Check sheet for the modelled part. Datum: model origin and axes. Units: mm. A direction names the side the tool comes from. Round coordinates to 2 decimals unless told otherwise and drop trailing zeros. Loops run counter-clockwise (first coordinate to the right, second up) from the corner with the lowest first, then second, coordinate; pieces in that order, holes last. Notation, with made-up numbers: (46, 60) - (89, 60) arc R26 ccw to (89, 76) - close; hole circle Ø2 at (14, 61). An arc over 180 degrees is marked (long way). Put each result on its own line as item: value. Start each with the question number.
Item 1: Gauge pin test, flat ends, axial feed: pin 1 Ø1.5 at (x, y) = (1.5, 10) entering from -Z; pin 2 Ø12 at (y, z) = (3.5, 5.5) entering from -X; pin 3 Ø1.5 at (x, y) = (1, -4.5) entering from +Z; pin 4 Ø1 at (x, z) = (1.5, -12.5) entering from -Y. Record the tip position at first contact, or that the pin passes through.
Item 2: Draft check along Z on faces 1 (the flat face through (0, 0, -4)), 2 (the cylindrical face through (1.528, 20.147, 2.645)), 3 (the cylindrical face through (1.53, 7.79, -13.1)). Enter one of: pulls with the +Z half, pulls with the -Z half, needs draft (parallel to the pull), parting line crosses it, or undercut.
Item 3: Section check B-B, the plane z = 0. Record the cut outline in (x, y).
Item 4: Tool access check on faces 4 (the flat face through (3.099, 0, -4)), 5 (the flat face through (2, 10, 1.905)). Record the directions out of +Z, -Z, +X, -X, +Y, -Y that give a thin tool (end or side, any length) a straight path to the whole face; none if there is none.
Item 5: Section check C-C, the plane z = 13.5. Record the cut outline in (x, y).
Item 6: Material ranges on line 1 along Y through (x, z) = (1.3, -7); line 2 along Z through (x, y) = (0.85, 7.5) (3 decimals); line 3 along Y through (x, z) = (1.05, 8.5), recorded low to high.
Item 7: Section check D-D, the plane y = 13. Record the cut outline in (x, z) (3 decimals).
Item 8: Section check A-A, the plane x = 1.7. Record the cut outline in (y, z) (1 decimal).
from build123d import *

# Parameters (mm, degrees)
SKETCH2_R           = 20.32
SKETCH2_R_2         = 1.0795
BOSS_EXTRUDE5_DEPTH = 3.0988


with BuildPart() as part:
    # Sketch2 → Boss-Extrude5 (new body)
    with BuildSketch(Plane(origin=(0, 0, 0), x_dir=(0, 0, -1), z_dir=(1, 0, 0))):
        Circle(SKETCH2_R)
        with BuildLine():
            Line((-12.142210048, -9.210012766), (-3.125861344, -4.004421414))
            ThreePointArc((-3.125861344, -4.004421414), (0, -5.08), (3.125861344, -4.004421414))
            Line((3.125861344, -4.004421414), (12.142210048, -9.210012766))
            ThreePointArc((12.142210048, -9.210012766), (0, -15.24), (-12.142210048, -9.210012766))
        make_face(mode=Mode.SUBTRACT)
        with BuildLine():
            ThreePointArc((-14.047210048, -5.910455977), (-13.198227154, 7.62), (-1.905, 15.120468743))
            Line((-1.905, 15.120468743), (-1.905, 4.709286039))
            ThreePointArc((-1.905, 4.709286039), (-4.399409051, 2.54), (-5.030861344, -0.704864625))
            Line((-5.030861344, -0.704864625), (-14.047210048, -5.910455977))
        make_face(mode=Mode.SUBTRACT)
        Circle(SKETCH2_R_2, mode=Mode.SUBTRACT)
        with BuildLine():
            Line((1.905, 4.709286039), (1.905, 15.120468743))
            ThreePointArc((1.905, 15.120468743), (13.198227154, 7.62), (14.047210048, -5.910455977))
            Line((14.047210048, -5.910455977), (5.030861344, -0.704864625))
            ThreePointArc((5.030861344, -0.704864625), (4.399409051, 2.54), (1.905, 4.709286039))
        make_face(mode=Mode.SUBTRACT)
    extrude(amount=BOSS_EXTRUDE5_DEPTH)


solid = part.part
Check result:
1. pin 1: z = -18.09
1. pin 2: x = 0
1. pin 3: z = 19.97
1. pin 4: y = -16.4
2. face 1: needs draft
2. face 2: parting line crosses it
2. face 3: undercut
3. outline: (0, -20.32) - (3.1, -20.32) - (3.1, -15.24) - (0, -15.24) - close; (0, -5.08) - (3.1, -5.08) - (3.1, -1.08) - (0, -1.08) - close; (0, 1.08) - (3.1, 1.08) - (3.1, 20.32) - (0, 20.32) - close
4. face 4: +Z, -Z, +X, +Y, -Y
4. face 5: +X, -X
5. outline: (0, -15.19) - (3.1, -15.19) - (3.1, -5.59) - (0, -5.59) - close; (0, 7.07) - (3.1, 7.07) - (3.1, 15.19) - (0, 15.19) - close
6. line 1: -19.08 to -13.54, -6.24 to -1.84, 13.54 to 19.08
6. line 2: -18.885 to -13.267, -1.905 to 1.905, 13.267 to 18.885
6. line 3: -18.46 to -12.65, -7.11 to -2.71, 12.65 to 18.46
7. outline: (0, -15.617) - (3.099, -15.617) - (3.099, -7.953) - (0, -7.953) - close; (0, -1.905) - (3.099, -1.905) - (3.099, 1.905) - (0, 1.905) - close; (0, 7.953) - (3.099, 7.953) - (3.099, 15.617) - (0, 15.617) - close
8. outline: circle Ø40.6 at (0, 0); hole (-9.2, -12.1) - (-4, -3.1) arc R5.1 cw to (-4, 3.1) - (-9.2, 12.1) arc R15.2 ccw to start; hole (-5.9, -14) arc R15.2 ccw to (15.1, -1.9) - (4.7, -1.9) arc R5.1 cw to (-0.7, -5) - close; hole (-5.9, 14) - (-0.7, 5) arc R5.1 cw to (4.7, 1.9) - (15.1, 1.9) arc R15.2 ccw to start; hole circle Ø2.2 at (0, 0)
